from build123d import *

# Parameters (mm, degrees)
BASE_FLANGE1_DEPTH = 16
SKETCH6_R          = 7
SKETCH6_R_2        = 1.984375
CUT_EXTRUDE1_DEPTH = 10
SKETCH7_R          = 1.5875
CUT_EXTRUDE2_DEPTH = 10


# Sheet-metal steps are written as plain solids
with BuildPart() as part:
    # Sketch1 → Base-Flange1 (new, symmetric)
    with BuildSketch(Plane.XY):
        with BuildLine():
            Line((-76.2, 0), (-0.7366, 0))
            ThreePointArc((-0.7366, 0), (-0.215745145, 0.215745145), (0, 0.7366))
            Line((0, 0.7366), (0, 101.6))
            Line((0, 101.6), (0.7366, 101.6))
            Line((0.7366, 101.6), (0.7366, 0.7366))
            ThreePointArc((0.7366, 0.7366), (0.30510971, -0.30510971), (-0.7366, -0.7366))
            Line((-0.7366, -0.7366), (-76.2, -0.7366))
            Line((-76.2, -0.7366), (-76.2, 0))
        make_face()
    extrude(amount=BASE_FLANGE1_DEPTH, both=True)

    # Sketch6 → Cut-Extrude1 (cut)
    with BuildSketch(Plane.ZY):
        with Locations((16, 29.2634)):
            Circle(SKETCH6_R)
        with Locations((8, 19.2634)):
            Circle(SKETCH6_R_2)
        with Locations((8, 39.2634)):
            Circle(SKETCH6_R_2)
        with Locations((8, 74.2634)):
            Circle(SKETCH6_R_2)
        with Locations((-8, 19.2634)):
            Circle(SKETCH6_R_2)
        with Locations((-16, 29.2634)):
            Circle(SKETCH6_R)
        with Locations((-8, 39.2634)):
            Circle(SKETCH6_R_2)
        with Locations((-8, 74.2634)):
            Circle(SKETCH6_R_2)
    extrude(amount=-CUT_EXTRUDE1_DEPTH, mode=Mode.SUBTRACT)

    # Sketch7 → Cut-Extrude2 (cut)
    with BuildSketch(Plane(origin=(0, 0, 0), x_dir=(1, 0, 0), z_dir=(0, 1, 0))):
        with Locations(Location((-30.7366, 0, 0), (0, 0, 270))):
            Circle(SKETCH7_R)
        with Locations(Location((-55.7366, -7.5, 0), (0, 0, 270))):
            Circle(SKETCH7_R)
        with Locations(Location((-55.7366, 7.5, 0), (0, 0, 270))):
            Circle(SKETCH7_R)
    extrude(amount=-CUT_EXTRUDE2_DEPTH, mode=Mode.SUBTRACT)


solid = part.part
Part model, mm, in its own coordinate system. A direction names the side the tool comes from. Round coordinates to 2 decimals unless told otherwise and drop trailing zeros. Write each loop counter-clockwise with the first axis right and the second up, starting at its lowest first coordinate (ties: lowest second). Pieces come first, ordered by that corner, then holes. Notation, with made-up numbers: (5.5, 22) - (28.5, 22) arc R13 cw to (28.5, 29) - close; hole circle Ø6 at (20.25, 74). An arc over 180 degrees is marked (long way). Use CSV: the item, a comma, the result in double quotes.
Item 1: Tool access for faces 1 (the flat face through (0, 50, 0)), 2 (the flat face through (0.737, 52, 0)): list every direction of +Z, -Z, +X, -X, +Y, -Y with a clear straight run to the whole face (end or side of a thin tool).
Results list:
face 1,"+Z, -Z, -X, +Y"
face 2,"+Z, -Z, +X, +Y, -Y"
Item 2: Slice it at A-A, the plane z = 0. Write the cut outline in (x, y), then the cut area to 3 significant figures.
Results list:
outline,"(-76.2, -0.74) - (-32.32, -0.74) - (-32.32, 0) - (-76.2, 0) - close; (-29.15, -0.74) - (-0.74, -0.74) arc R1.47 ccw to (0.74, 0.74) - (0.74, 101.6) - (0, 101.6) - (0, 0.74) arc R0.74 cw to (-0.74, 0) - (-29.15, 0) - close"
area,"129 mm²"
Item 3: Slice it at D-D, the plane x = -22. Write the cut outline in (y, z).
Results list:
outline,"(-0.74, -16) - (0, -16) - (0, 16) - (-0.74, 16) - close"
Item 4: Slice it at B-B, the plane z = 7.5. Write the cut outline in (x, y), then the cut area to 3 significant figures.
Results list:
outline,"(-76.2, -0.74) - (-57.32, -0.74) - (-57.32, 0) - (-76.2, 0) - close; (-54.15, -0.74) - (-0.74, -0.74) arc R1.47 ccw to (0.74, 0.74) - (0.74, 17.34) - (0, 17.34) - (0, 0.74) arc R0.74 cw to (-0.74, 0) - (-54.15, 0) - close; (0, 21.18) - (0.74, 21.18) - (0.74, 37.34) - (0, 37.34) - close; (0, 41.18) - (0.74, 41.18) - (0.74, 72.34) - (0, 72.34) - close; (0, 76.18) - (0.74, 76.18) - (0.74, 101.6) - (0, 101.6) - close"
area,"120 mm²"
Item 5: Pull direction Y, two halves, no side cores. Call faces 3 (the flat face through (-39, 0, 0)), 4 (the cylindrical face through (0.363, 37.326, 7.57)), 5 (the cylindrical face through (-56.34, -0.36, 8.97)): pulls with the +Y half, pulls with the -Y half, needs draft (parallel to the pull), parting line crosses it, or undercut.
Results list:
face 3,"pulls with the +Y half"
face 4,"undercut"
face 5,"needs draft"
Item 6: Slice it at C-C, the plane z = -12. Write the cut outline in (x, y).
Results list:
outline,"(-76.2, -0.74) - (-0.74, -0.74) arc R1.47 ccw to (0.74, 0.74) - (0.74, 23.52) - (0, 23.52) - (0, 0.74) arc R0.74 cw to (-0.74, 0) - (-76.2, 0) - close; (0, 35.01) - (0.74, 35.01) - (0.74, 101.6) - (0, 101.6) - close"
Item 7: Flat gauge pins, fed straight in: P1, Ø4.5, axis at y = 74.26, z = 8, coming from the -X side; P2, Ø12, axis at x = -51, z = 0.5, coming from the +Y side. Where does each tip first touch, or does it go through?
Results list:
P1,"stops at x = 0"
P2,"stops at y = 0"
Item 8: Wall check: L1, parallel to Y at x = 0.3, z = 8; L2, parallel to X at y = 48.5, z = -3.5; L3, parallel to Y at x = -36, z = 2. Give the ranges that are in metal, low to high.
Results list:
L1,"y = -0.31 to 17.28, 21.25 to 37.28, 41.25 to 72.28, 76.25 to 101.6"
L2,"x = 0 to 0.74"
L3,"y = -0.74 to 0"
